Autodesk Fusion 360 part; units mm, degrees
sketch "スケッチ1" plane through (0, 0, 0) normal (0, 0, 1) x (1, 0, 0)
  line L0 (-17.5, 170) -> (17.5, 170)
  line L1 (17.5, 170) -> (17.5, 0)
  line L2 (17.5, 0) -> (-17.5, 0)
  line L3 (-17.5, 0) -> (-17.5, 170)
  circle A0 centre (12, 5) radius 2
  circle A1 centre (-12, 5) radius 2
  line L4 (12, 5) -> (-12, 5) construction
  circle A2 centre (0, 160) radius 2.25
  dimension "d1" = 170
  dimension "d2" = 35
  dimension "d3" = 4
  dimension "d4" = 4
  dimension "d5" = 24
  dimension "d6" = 5
  dimension "d7" = 5.5
  dimension "d8" = 4.5
  dimension "d9" = 155
extrude "押し出し1" add sketch "スケッチ1" along normal blind 2 makes body 1
sketch "スケッチ2" plane through (0, 0, 2) normal (0, 0, 1) x (-1, 0, 0)
  circle A0 centre (-12, -5) radius 2
  circle A1 centre (0, -160) radius 2.25
  circle A2 centre (12, -5) radius 2
  line L0 (17.5, 0) -> (-17.5, 0)
  line L1 (-17.5, 0) -> (-17.5, -170)
  line L2 (-17.5, -170) -> (17.5, -170)
  line L3 (17.5, -170) -> (17.5, 0)
  line L4 (-7, -170) -> (-17.5, -170)
  line L5 (-17.5, -170) -> (-17.5, -10)
  line L6 (-17.5, -10) -> (-7, -10)
  line L7 (-7, -10) -> (-7, -170)
  line L8 (17.5, -170) -> (7, -170)
  line L9 (7, -170) -> (7, -10)
  line L10 (7, -10) -> (17.5, -10)
  line L11 (17.5, -10) -> (17.5, -170)
  dimension "d12" = 10.5
  dimension "d13" = 10
  dimension "d14" = 10.5
  dimension "d15" = 10
extrude "押し出し2" cut sketch "スケッチ2" against normal blind 2 contours L2 L3 L8 L9 L10 L11 | L1 L2 L4 L5 L6 L7 bodies 1
sketch "スケッチ3" plane through (7, 0, 0) normal (1, 0, 0) x (0, 1, 0)
  line L0 (170, 2) -> (10, 2)
  line L1 (10, 2) -> (10, 0)
  line L2 (10, 0) -> (170, 0)
  line L3 (170, 0) -> (170, 2)
  line L4 (10, 15) -> (103, 15)
  line L5 (103, 15) -> (103, 0)
  line L6 (103, 0) -> (10, 0)
  line L7 (10, 0) -> (10, 15)
  dimension "d18" = 15
  dimension "d19" = 93
extrude "押し出し3" add sketch "スケッチ3" along normal blind 2 separate body contours L0 L1 L2 L5 L6 L7 | L0 L4 L5 L7 makes body 2
sketch "スケッチ4" plane through (-7, 0, 0) normal (-1, 0, 0) x (0, -1, 0)
  line L0 (-10, 2) -> (-170, 2)
  line L1 (-170, 2) -> (-170, 0)
  line L2 (-170, 0) -> (-10, 0)
  line L3 (-10, 0) -> (-10, 2)
  line L4 (-10, 15) -> (-103, 15)
  line L5 (-103, 15) -> (-103, 0)
  line L6 (-103, 0) -> (-10, 0)
  line L7 (-10, 0) -> (-10, 15)
  line L8 (-103, 15) -> (-103, 0)
  line L9 (-10, 0) -> (-10, 15)
  line L10 (-10, 15) -> (-103, 15)
extrude "押し出し4" add sketch "スケッチ4" along normal blind 2 separate body contours L0 L2 L3 L5 L6 L7 L8 L9 | L0 L4 L5 L7 L8 L9 L10 makes body 3
sketch "スケッチ5" plane through (0, 0, 2) normal (0, 0, 1) x (-1, 0, 0)
  line L0 (7, -170) -> (7, -10)
  line L1 (7, -10) -> (17.5, -10)
  line L2 (17.5, -10) -> (17.5, 0)
  line L3 (17.5, 0) -> (-17.5, 0)
  line L4 (-17.5, 0) -> (-17.5, -10)
  line L5 (-17.5, -10) -> (-7, -10)
  line L6 (-7, -10) -> (-7, -170)
  line L7 (-7, -170) -> (7, -170)
  circle A0 centre (12, -5) radius 2
  circle A1 centre (0, -160) radius 2.25
  circle A2 centre (-12, -5) radius 2
  line L8 (-7, -170) -> (-10, -170)
  line L9 (-10, -170) -> (-10, -103)
  line L10 (-10, -103) -> (-7, -103)
  line L11 (-7, -103) -> (-7, -170)
  line L12 (-7, -103) -> (-9, -103)
  line L13 (7, -170) -> (13, -170)
  line L14 (13, -170) -> (13, -103)
  line L15 (13, -103) -> (7, -103)
  line L16 (7, -103) -> (7, -170)
  line L17 (7, -103) -> (9, -103)
  dimension "d24" = 3
  dimension "d25" = 6
extrude "押し出し5" add sketch "スケッチ5" against normal blind 2 contours L0 L13 L14 L15 L16 L17 | L6 L8 L9 L10 L11 L12 bodies 1 2 3
sketch "スケッチ10" plane through (-13, 0, 0) normal (-1, 0, 0) x (0, -1, 0)
  line L0 (-103, 2) -> (-170, 2)
  line L1 (-170, 2) -> (-170, 0)
  line L2 (-170, 0) -> (-103, 0)
  line L3 (-103, 0) -> (-103, 2)
  line L4 (-103, 0) -> (-170, 0)
  line L5 (-170, 0) -> (-170, 15)
  line L6 (-170, 15) -> (-103, 15)
  line L7 (-103, 15) -> (-103, 0)
  point P0 (-103, 15)
extrude "押し出し8" add sketch "スケッチ10" along normal blind 2 separate body makes body 4
sketch "スケッチ11" plane through (10, 0, 0) normal (1, 0, 0) x (0, 1, 0)
  line L0 (170, 2) -> (103, 2)
  line L1 (103, 2) -> (103, 0)
  line L2 (103, 0) -> (170, 0)
  line L3 (170, 0) -> (170, 2)
  line L4 (103, 0) -> (170, 0)
  line L5 (170, 0) -> (170, 15)
  line L6 (170, 15) -> (103, 15)
  line L7 (103, 15) -> (103, 0)
  line L8 (103, 15) -> (10, 15)
extrude "押し出し9" add sketch "スケッチ11" along normal blind 2 separate body makes body 5
sketch "スケッチ12" plane through (0, 103, 0) normal (0, -1, 0) x (1, 0, 0)
  line L0 (-13, 0) -> (-13, 15)
  line L1 (-13, 15) -> (-15, 15)
  line L2 (-15, 15) -> (-15, 0)
  line L3 (-15, 0) -> (-13, 0)
  line L4 (-15, 15) -> (-7, 15)
  line L5 (-7, 15) -> (-7, 0)
  line L6 (-7, 0) -> (-15, 0)
  line L7 (-15, 0) -> (-15, 15)
  line L8 (-7, 2) -> (-7, 15)
  line L9 (17.5, 0) -> (-17.5, 0)
  line L10 (7, 15) -> (12, 15)
  line L11 (12, 15) -> (12, 0)
  line L12 (12, 0) -> (7, 0)
  line L13 (7, 0) -> (7, 15)
  line L14 (12, 15) -> (12, 0)
  line L15 (7, 2) -> (7, 15)
  line L16 (10, 15) -> (12, 15)
extrude "押し出し10" add sketch "スケッチ12" along normal blind 2 bodies 1 4 5
sketch "スケッチ13" plane through (0, 10, 0) normal (0, 1, 0) x (-1, 0, 0)
  line L0 (-9, 0) -> (-9, 2)
  line L1 (-9, 2) -> (-17.5, 2)
  line L2 (-17.5, 2) -> (-17.5, 0)
  line L3 (-17.5, 0) -> (-9, 0)
  line L4 (-17.5, 0) -> (-7, 0)
  line L5 (-7, 0) -> (-7, 15)
  line L6 (-7, 15) -> (-17.5, 15)
  line L7 (-17.5, 15) -> (-17.5, 0)
  line L8 (7, 15) -> (17.5, 15)
  line L9 (17.5, 15) -> (17.5, 0)
  line L10 (17.5, 0) -> (7, 0)
  line L11 (7, 0) -> (7, 15)
  point P0 (-7, 15)
  point P1 (7, 15)
  point P2 (17.5, 0)
extrude "押し出し11" add sketch "スケッチ13" along normal blind 2 bodies 1
sketch "スケッチ14" plane through (0, 0, 2) normal (0, 0, 1) x (-1, 0, 0)
  line L0 (7, -103) -> (7, -10)
  line L1 (7, -10) -> (17.5, -10)
  line L2 (17.5, -10) -> (17.5, 0)
  line L3 (17.5, 0) -> (-17.5, 0)
  line L4 (-17.5, 0) -> (-17.5, -10)
  line L5 (-17.5, -10) -> (-7, -10)
  line L6 (-7, -10) -> (-7, -103)
  line L7 (-7, -103) -> (-10, -103)
  line L8 (-10, -103) -> (-10, -170)
  line L9 (-10, -170) -> (13, -170)
  line L10 (13, -170) -> (13, -103)
  line L11 (13, -103) -> (7, -103)
  circle A0 centre (12, -5) radius 2
  circle A1 centre (0, -160) radius 2.25
  circle A2 centre (-12, -5) radius 2
  line L12 (7, -103) -> (-7, -103)
  line L13 (-7, -103) -> (-7, -10)
  line L14 (-7, -10) -> (7, -10)
  line L15 (7, -10) -> (7, -103)
extrude "押し出し12" add sketch "スケッチ14" along normal blind 2 contours L0 L6 L12 L13 L14 L15 bodies 1
sketch "スケッチ15" plane through (0, 0, 2) normal (0, 0, 1) x (-1, 0, 0)
  circle A0 centre (0, -160) radius 2.25
  line L0 (13, -103) -> (-10, -103)
  line L1 (-10, -103) -> (-10, -170)
  line L2 (-10, -170) -> (13, -170)
  line L3 (13, -170) -> (13, -103)
  circle A1 centre (0, -160) radius 4
  dimension "d43" = 8
extrude "押し出し13" add sketch "スケッチ15" along normal blind 5 contours A1 bodies 1
sketch "スケッチ19" plane through (0, 0, 0) normal (0, 0, -1) x (1, 0, 0)
  line L0 (-9, -12) -> (-9, -101)
  line L1 (-9, -101) -> (-15, -101)
  line L2 (-15, -101) -> (-15, -170)
  line L3 (-15, -170) -> (12, -170)
  line L4 (12, -170) -> (12, -101)
  line L5 (12, -101) -> (9, -101)
  line L6 (9, -101) -> (9, -12)
  line L7 (9, -12) -> (17.5, -12)
  line L8 (17.5, -12) -> (17.5, 0)
  line L9 (17.5, 0) -> (-17.5, 0)
  line L10 (-17.5, 0) -> (-17.5, -12)
  line L11 (-17.5, -12) -> (-9, -12)
  circle A0 centre (-12, -5) radius 2
  circle A1 centre (0, -160) radius 2.25
  circle A2 centre (12, -5) radius 2
  line L12 (19, -12) -> (-19, -12)
  line L13 (-19, -12) -> (-19, 118)
  line L14 (-19, 118) -> (19, 118)
  line L15 (19, 118) -> (19, -12)
  line L16 (0, -1.75) -> (0, -22.5)
  dimension "d53" = 130
  dimension "d54" = 38
extrude "押し出し16" add sketch "スケッチ19" against normal blind 2 contours L8 L9 L10 L12 L13 L14 L15 bodies 1
sketch "スケッチ21" plane through (0, 0, 2) normal (0, 0, 1) x (-1, 0, 0)
  line L0 (-17.5, -10) -> (17.5, -10)
  line L1 (17.5, -10) -> (17.5, -12)
  line L2 (17.5, -12) -> (19, -12)
  line L3 (19, -12) -> (19, 118)
  line L4 (19, 118) -> (-19, 118)
  line L5 (-19, 118) -> (-19, -12)
  line L6 (-19, -12) -> (-17.5, -12)
  line L7 (-17.5, -12) -> (-17.5, -10)
  circle A0 centre (12, -5) radius 2
  circle A1 centre (-12, -5) radius 2
  line L8 (19, -12) -> (17, -12)
  line L9 (17, -12) -> (17, 98)
  line L10 (17, 98) -> (19, 98)
  line L11 (19, 98) -> (19, -12)
  line L12 (-19, -12) -> (-17, -12)
  line L13 (-17, -12) -> (-17, 98)
  line L14 (-17, 98) -> (-19, 98)
  line L15 (-19, 98) -> (-19, -12)
  dimension "d59" = 110
  dimension "d60" = 110
  dimension "d61" = 2
  dimension "d62" = 2
extrude "押し出し17" add sketch "スケッチ21" along normal blind 15 contours L0 L5 L6 L7 L12 L13 L14 L15 | L0 L1 L2 L3 L8 L9 L10 L11 bodies 1
sketch "スケッチ22" plane through (0, 0, 2) normal (0, 0, 1) x (-1, 0, 0)
  circle A0 centre (-12, -5) radius 2
  circle A1 centre (12, -5) radius 2
  line L0 (-19, 98) -> (-17, 98)
  line L1 (-17, 98) -> (-17, -10)
  line L2 (-17, -10) -> (17, -10)
  line L3 (17, -10) -> (17, 98)
  line L4 (17, 98) -> (19, 98)
  line L5 (19, 98) -> (19, 118)
  line L6 (19, 118) -> (-19, 118)
  line L7 (-19, 118) -> (-19, 98)
  line L8 (-19, 118) -> (19, 118)
  line L9 (19, 118) -> (19, 98)
  line L10 (19, 98) -> (-19, 98)
  line L11 (-19, 98) -> (-19, 118)
extrude "押し出し18" add sketch "スケッチ22" along normal blind 15 contours L0 L4 L5 L6 L7 L8 L9 L10 L11 bodies 1
sketch "スケッチ25" plane through (0, -118, 0) normal (0, -1, 0) x (1, 0, 0)
  line L0 (-19, 0) -> (19, 0)
  line L1 (19, 0) -> (19, 17)
  line L2 (19, 17) -> (-19, 17)
  line L3 (-19, 17) -> (-19, 0)
  circle A0 centre (0, 17) radius 9
  dimension "d69" = 18
extrude "押し出し19" cut sketch "スケッチ25" against normal up to surface (20 mm away) contours L2 A0 picked at (-1.096, 14.2074) bodies 1
ref_plane "作業平面3" through (0, -109, 8.5) normal (0, -1, 0) x (1, 0, 0)
sketch "スケッチ26" plane through (0, -109, 8.5) normal (0, -1, 0) x (1, 0, 0)
  line L0 (-16, 8.5) -> (16, 8.5)
  line L1 (16, 8.5) -> (16, -2.5)
  line L2 (16, -2.5) -> (-16, -2.5)
  line L3 (-16, -2.5) -> (-16, 8.5)
  line L4 (9, 8.5) -> (19, 8.5)
  line L5 (0, -6.75) -> (0, 14)
  dimension "d73" = 32
  dimension "d74" = 11
extrude "押し出し20" cut sketch "スケッチ26" against normal blind 2.25 bodies 1
sketch "スケッチ29" plane through (0, 0, 17) normal (0, 0, 1) x (-1, 0, 0)
  line L0 (16, 106.75) -> (9, 106.75)
  line L1 (9, 106.75) -> (9, 98)
  line L2 (9, 98) -> (17, 98)
  line L3 (17, 98) -> (17, -10)
  line L4 (17, -10) -> (17.5, -10)
  line L5 (17.5, -10) -> (17.5, -12)
  line L6 (17.5, -12) -> (19, -12)
  line L7 (19, -12) -> (19, 118)
  line L8 (19, 118) -> (9, 118)
  line L9 (9, 118) -> (9, 109)
  line L10 (9, 109) -> (16, 109)
  line L11 (16, 109) -> (16, 106.75)
  line L12 (15, 102.75) -> (-15, 102.75) construction
  line L13 (-15, 102.75) -> (-15, 113) construction
  line L14 (-15, 113) -> (15, 113) construction
  line L15 (15, 113) -> (15, 102.75) construction
  line L16 (-16, 106.75) -> (-16, 109) construction
  circle A0 centre (15, 102.75) radius 1.75
  circle A1 centre (15, 113) radius 1.75
  circle A2 centre (-15, 113) radius 1.75
  circle A3 centre (-15, 102.75) radius 1.75
  dimension "d85" = 1
  dimension "d86" = 4
  dimension "d87" = 4
  dimension "d88" = 1
  dimension "d89" = 3.5
  dimension "d90" = 3.5
  dimension "d91" = 3.5
  dimension "d92" = 3.5
extrude "押し出し22" cut sketch "スケッチ29" against normal blind 10 contours A0 | A1 | A2 | A3 bodies 1
Work out the finished part from the listing and answer in its coordinate system (mm). A direction names the side the tool comes from. Round coordinates to 2 decimals unless told otherwise and drop trailing zeros. Write each loop counter-clockwise with the first axis right and the second up, starting at its lowest first coordinate (ties: lowest second). Pieces come first, ordered by that corner, then holes.
1) Straight lines are drawn through the part: line 1 (Y direction, x = -7.5, z = 10.5); line 2 (Y direction, x = 10.5, z = 9.5); line 3 (X direction, y = -56, z = 15). For each, find the intervals that lie inside material, in ascending order.
2) Given pin 1 Ø1 at (x, z) = (-9, 14.5) entering from +Y; pin 2 Ø1.8 at (x, y) = (-15.5, -103) entering from +Z; pin 3 Ø10 at (y, z) = (108.5, 7) entering from -X, each flat-ended and moving along its own axis, determine where each tip first touches the part or whether it passes through.
3) A cutting plane is placed at B-B (z = 10.5). Give the number of separate pieces and of enclosed holes in the cut face, plus the area to 3 significant figures.
4) A cutting plane is placed at C-C (y = -12.5). Give the vertices of the cut face in (x, z), plus the area to 3 significant figures.
5) A tool of negligible diameter and unlimited length cuts with its end or side. For faces 4 (the flat face through (0, 10, 3)), 5 (the flat face through (12, 135, 8)), 6 (the flat face through (7, 56, 10)), 7 (the cylindrical face through (0, -114, 8)), from which of +Z, -Z, +X, -X, +Y, -Y can it reach the whole face along a straight path? Write none if from no direction.
6) The mould has two halves that part along X. Classify faces 1 (the flat face through (-9, 57, 8)), 2 (the flat face through (-12, 101, 8)), 3 (the cylindrical face through (-0.148, 162.245, 3.451)): pulls with the +X half, pulls with the -X half, needs draft (parallel to the pull), parting line crosses it, or undercut.
7) A cutting plane is placed at A-A (y = 111.5). Give the vertices of the cut face in (x, z).
Completed:
1. line 1: y = -118 to -109, -106.75 to -98, 10 to 103
1. line 2: y = -118 to -109, -106.75 to -98, 10 to 12, 101 to 170
1. line 3: x = -19 to -17, 17 to 19
2. pin 1: stops at y = 103
2. pin 2: stops at z = 7
2. pin 3: stops at x = -15
3. separate pieces: 2
3. enclosed holes: 4
3. area: 1,560 mm2
4. outline: (-19, 0) - (19, 0) - (19, 17) - (17, 17) - (17, 2) - (-17, 2) - (-17, 17) - (-19, 17) - close
4. area: 136 mm2
5. face 4: +Z
5. face 5: +Z, -Z, +X, +Y
5. face 6: +Z, +Y
5. face 7: +Z, -Y
6. face 1: pulls with the -X half
6. face 2: needs draft
6. face 3: undercut
7. outline: (-15, 0) - (12, 0) - (12, 15) - (10, 15) - (10, 2) - (-13, 2) - (-13, 15) - (-15, 15) - close
